The figure shows three views and two pictorial views of one solid part (mm, origin at its lowest corner). Answer the questions. Give positions to 0.01 mm unless a question says otherwise; leave off trailing zeros. Loops run counter-clockwise (first coordinate to the right, second up) from the corner with the lowest first, then second, coordinate; pieces in that order, holes last.
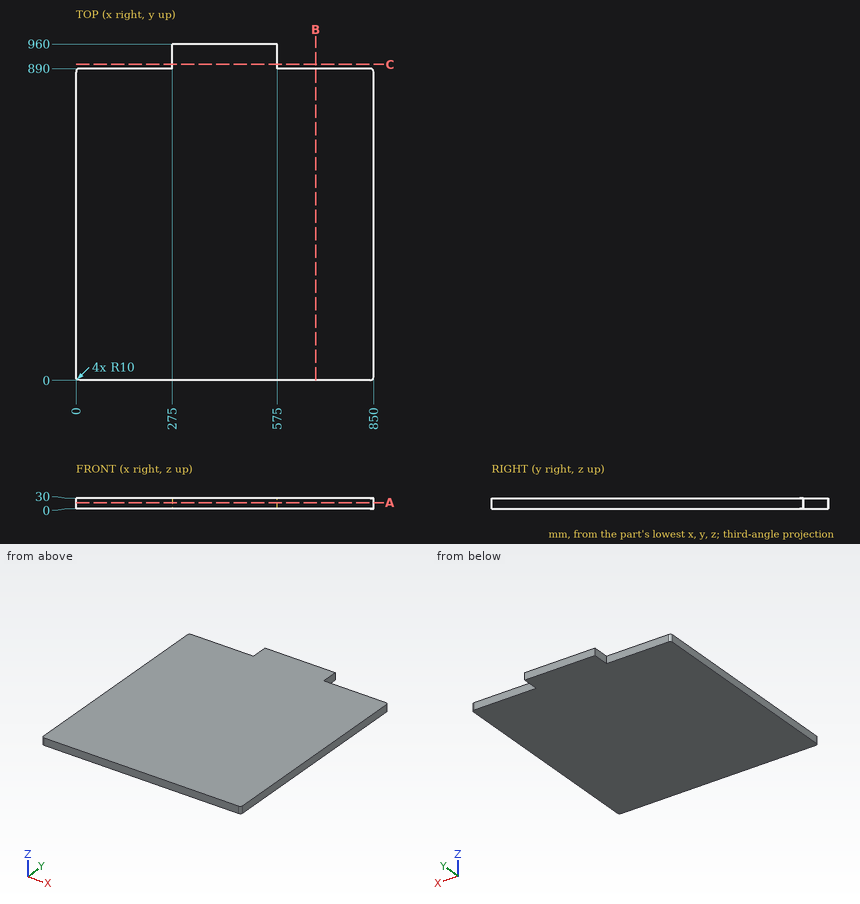
Q1. Section C-C on y = 902 is taken. Give the vertices of the cut face in (x, z), plus the area to 3 significant figures.
Q2. Given pin 1 (15 mm diameter, centred on y = 940, z = 12, fed in from +X); pin 2 (9 mm diameter, centred on x = 189.5, z = 10.5, fed in from +Y); pin 3 (15 mm diameter, centred on y = 933, z = 15.5, fed in from -X), each flat-ended and moving along its own axis, determine where each tip first touches the part or whether it passes through.
Q3. Section A-A on z = 17.5 is taken. Give the vertices of the cut face in (x, y).
Q4. Section B-B on x = 684 is taken. Give the vertices of the cut face in (y, z), plus the area to 3 significant figures.
Q5. Consider line 1 along Y through (x, z) = (627, 2.5). Determine where the line is inside the solid, lowest interval first.
Check result:
1. outline: (275, 0) - (575, 0) - (575, 30) - (275, 30) - close
1. area: 9,000 mm2
2. pin 1: stops at x = 575
2. pin 2: stops at y = 890
2. pin 3: stops at x = 275
3. outline: (0, 10) arc R10 ccw to (10, 0) - (840, 0) arc R10 ccw to (850, 10) - (850, 880) arc R10 ccw to (840, 890) - (575, 890) - (575, 960) - (275, 960) - (275, 890) - (10, 890) arc R10 ccw to (0, 880) - close
4. outline: (0, 0) - (890, 0) - (890, 30) - (0, 30) - close
4. area: 26,700 mm2
5. line 1: y = 0 to 890
